Geometry check sheet. Reference: the model listing, model coordinates, mm. Face numbers are marked on the shaded views. A direction names the side the tool comes from. Coordinates: 2 decimals unless noted, no trailing zeros. Order: outer loops, then holes, each group sorted by start corner. A loop starts at its lowest first (then second) coordinate and runs counter-clockwise, first axis right, second up. Notation, with made-up numbers: M 57.5,41 L 92.5,41 A4 ccw 92.5,46 Z; hole C 81.25,46.25 d8. An arc over 180 degrees is marked long. One line per item, written item: value. Start each with the question number.
1) Access from +Z, -Z, +X, -X, +Y, -Y to the whole of each face (thin tool, end or side, straight path). Record for the marked faces 5 and 6.
2) Draft check along X on the marked faces 1, 2, 3 and 4. Enter one of: pulls with the +X half, pulls with the -X half, needs draft (parallel to the pull), parting line crosses it, or undercut.
3) Sectioned sample at B-B, the plane x = -25. Enter the section's corners in (y, z), then the cut area to 3 significant figures.
4) Sectioned sample at C-C, the plane z = 2.5. Enter the section's corners in (x, y).
5) Thickness scan on L1, parallel to Y at x = -25, z = -6.25; L2, parallel to Z at x = -27, y = 9.5; L3, parallel to Y at x = -42, z = 5. Record the ranges inside material, lowest first. Write a range as from..to.
6) Sectioned sample at A-A, the plane y = 35. Enter the section's corners in (x, z).
7) Sectioned sample at D-D, the plane z = -17.75. Enter the section's corners in (x, y), then the cut area to 3 significant figures.
8) Go/stop test with flat-tipped pins: P1, Ø5, axis at x = -28, y = 6, coming from the -Z side; P2, Ø8, axis at y = 5, z = 4, coming from the +X side; P3, Ø1.5, axis at x = -30, z = -16.5, coming from the -Y side. Record where each tip stops, or that it passes through.
```python
from build123d import *

# Parameters (mm, degrees)
BOSS_EXTRUDE1_DEPTH = 10
SKETCH2_W           = 50
SKETCH2_H           = 85
BOSS_EXTRUDE2_DEPTH = 20
SKETCH3_R           = 6
CUT_EXTRUDE1_DEPTH  = 20


with BuildPart() as part:
    # Sketch1 → Boss-Extrude1 (new body)
    with BuildSketch(Plane.XY):
        Polygon((-10, 0), (-40, 0), (-40, 10), (-50, 10), (-50, 95), (-40, 95), (-40, 100), (-10, 100), (-10, 95), (0, 95), (0, 10), (-10, 10), align=None)
    extrude(amount=BOSS_EXTRUDE1_DEPTH)

    # Sketch2 → Boss-Extrude2 (add)
    with BuildSketch(Plane(origin=(0, 0, 0), x_dir=(-1, 0, 0), z_dir=(0, 0, -1))):
        with Locations((25, 52.5)):
            Rectangle(SKETCH2_W, SKETCH2_H)
    extrude(amount=BOSS_EXTRUDE2_DEPTH)

    # Sketch3 → Cut-Extrude1 (cut)
    with BuildSketch(Plane(origin=(0, 0, -20), x_dir=(-1, 0, 0), z_dir=(0, 0, -1))):
        with Locations((25, 35)):
            Circle(SKETCH3_R)
    extrude(amount=-CUT_EXTRUDE1_DEPTH, mode=Mode.SUBTRACT)


solid = part.part
```
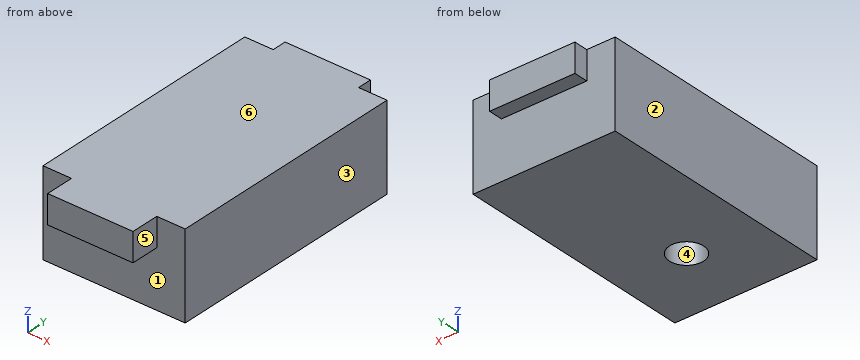
Final values:
1. face 5: +Z, -Z, +X, -Y
1. face 6: +Z, +X, -X, +Y, -Y
2. face 1: needs draft
2. face 2: pulls with the -X half
2. face 3: pulls with the +X half
2. face 4: undercut
3. outline: M 0,0 L 10,0 L 10,-20 L 29,-20 L 29,0 L 41,0 L 41,-20 L 95,-20 L 95,0 L 100,0 L 100,10 L 0,10 Z
3. area: 2,460 mm^2
4. outline: M -50,10 L -40,10 L -40,0 L -10,0 L -10,10 L 0,10 L 0,95 L -10,95 L -10,100 L -40,100 L -40,95 L -50,95 Z
5. L1: y = 10..29, 41..95
5. L2: z = 0..10
5. L3: y = 10..95
6. outline: M -50,-20 L -31,-20 L -31,0 L -19,0 L -19,-20 L 0,-20 L 0,10 L -50,10 Z
7. outline: M -50,10 L 0,10 L 0,95 L -50,95 Z; hole C -25,35 d12
7. area: 4,140 mm^2
8. P1: stops at z = 0
8. P2: stops at x = -10
8. P3: stops at y = 10
